from build123d import *

# Parameters (mm, degrees)
F0_R     = 20
F1_DEPTH = 17
F2_R     = 5
F3_DEPTH = 30.001
F4_DEPTH = 12.5
F0_R_2   = 5
F5_DEPTH = 14.5


# Not quite as in the source:
# - a feature names something its author has since deleted; it is built from what else it names


with BuildPart() as f1:
    # F0 (on Front) → F1 (new body, symmetric)
    with BuildSketch(Plane.XZ):
        with BuildLine():
            ThreePointArc((-22.5, 19.843134833), (-10.6066017178, -28.0624304008), (30, 0))
            ThreePointArc((30, 0), (28.0624304008, 10.6066017178), (22.5, 19.843134833))
            ThreePointArc((22.5, 19.843134833), (0, 30), (-22.5, 19.843134833))
        make_face()
        Circle(F0_R, mode=Mode.SUBTRACT)
    extrude(amount=F1_DEPTH, both=True)

    # F2 (on Right) → F3 (cut, through all)
    with BuildSketch(Plane.YZ):
        Circle(F2_R)
    extrude(amount=F3_DEPTH, mode=Mode.SUBTRACT)

    # F0 (on Front) → F4 (cut, symmetric)
    with BuildSketch(Plane.XZ):
        with BuildLine():
            ThreePointArc((6, 79.5607177772), (0, 78.5), (-6, 79.5607177772))
            Line((-6, 79.5607177772), (-6, 73.6))
            Line((-6, 73.6), (6, 73.6))
            Line((6, 73.6), (6, 79.5607177772))
        make_face()
    extrude(amount=F4_DEPTH, both=True, mode=Mode.SUBTRACT)

    # F0 (on Front) → F5 (join, symmetric)
    with BuildSketch(Plane.XZ):
        with BuildLine():
            ThreePointArc((-22.5, 19.843134833), (0, 30), (22.5, 19.843134833))
            Line((22.5, 19.843134833), (22.5, 166))
            Line((22.5, 166), (-22.5, 166))
            Line((-22.5, 166), (-22.5, 19.843134833))
        make_face()
        with BuildLine():
            ThreePointArc((-6, 79.5607177772), (-10.0312013239, 110.3396303997), (17.5, 96))
            ThreePointArc((17.5, 96), (14.3396303997, 85.9687986761), (6, 79.5607177772))
            Line((6, 79.5607177772), (6, 73.6))
            Line((6, 73.6), (-6, 73.6))
            Line((-6, 73.6), (-6, 79.5607177772))
        make_face(mode=Mode.SUBTRACT)
        with Locations((0, 140)):
            Circle(F0_R_2, mode=Mode.SUBTRACT)
    extrude(amount=F5_DEPTH, both=True)


solid = f1.part
Work out the finished part from the listing and answer in its coordinate system (mm). A direction names the side the tool comes from. Give positions to 0.01 mm unless a question says otherwise; leave off trailing zeros. Write each loop counter-clockwise with the first axis right and the second up, starting at its lowest first coordinate (ties: lowest second). Pieces come first, ordered by that corner, then holes. Notation, with made-up numbers: (85.5, 43.5) - (114.5, 43.5) arc R8 ccw to (114.5, 58.5) - close; hole circle Ø2 at (-35.75, 10.25). An arc over 180 degrees is marked (long way). One line per item, written item: value. Start each with the question number.
1. Consider probe 1 along Z at (x, y) = (0, 1); probe 2 along Y at (x, z) = (27, 0); probe 3 along Z at (x, y) = (5.5, 2). Determine where each line is inside the solid, lowest interval first.
2. For faces 4 (the flat face through (20, -17, -6)), 5 (the cylindrical face through (25, -5, 0)), 6 (the flat face through (-6, 0, 77)), 7 (the flat face through (22.5, 0, 92)), determine the directions among +Z, -Z, +X, -X, +Y, -Y from which every point of the face is accessible in a straight line to the end or side of a thin tool.
3. Find section D-D (z = 96). Write down the section's boundary in (x, y).
4. For a pull along X with two mould halves and no side action, classify faces 1 (the flat face through (20, 17, -6)), 2 (the flat face through (6, 0, 77)), 3 (the flat face through (-22.5, 0, 94)) as +X half, -X half, draft (parallel to the pull), parting line (faces both ways), or undercut.
5. Find section A-A (z = 0). Write down the section's boundary in (x, y).
6. Given pin 1 (4 mm diameter, centred on x = 5.5, z = 59.5, fed in from +Y); pin 2 (5 mm diameter, centred on y = -5.5, z = 28, fed in from -X); pin 3 (11.5 mm diameter, centred on x = 0, z = 140, fed in from -Y), each flat-ended and moving along its own axis, determine where each tip first touches the part or whether it passes through.
7. Find section B-B (x = 0). Write down the section's boundary in (y, z), then the cut area to 3 significant figures.
8. Find section C-C (y = 7). Write down the section's boundary in (x, z), then the cut area to 3 significant figures.
Geometry results:
1. probe 1: -30 to -20, 20 to 73.6, 113.5 to 135, 145 to 166
1. probe 2: -17 to -5, 5 to 17
1. probe 3: -29.49 to -19.23, 19.23 to 73.6, 112.61 to 166
2. face 4: +Z, -Z, +X, -X, -Y
2. face 5: +X
2. face 6: +Y, -Y
2. face 7: +Z, +X, +Y, -Y
3. outline: (-22.5, -14.5) - (-17.5, -14.5) - (-17.5, 14.5) - (-22.5, 14.5) - close; (17.5, -14.5) - (22.5, -14.5) - (22.5, 14.5) - (17.5, 14.5) - close
4. face 1: draft
4. face 2: undercut
4. face 3: -X half
5. outline: (-30, -17) - (-20, -17) - (-20, 17) - (-30, 17) - close; (20, -17) - (30, -17) - (30, -5) - (20, -5) - close; (20, 5) - (30, 5) - (30, 17) - (20, 17) - close
6. pin 1: y = 14.5
6. pin 2: x = -22.5
6. pin 3: y = -14.5
7. outline: (-17, -30) - (17, -30) - (17, -20) - (-17, -20) - close; (-17, 20) - (17, 20) - (17, 30) - (14.5, 30) - (14.5, 73.6) - (-14.5, 73.6) - (-14.5, 30) - (-17, 30) - close; (-14.5, 113.5) - (14.5, 113.5) - (14.5, 135) - (-14.5, 135) - close; (-14.5, 145) - (14.5, 145) - (14.5, 166) - (-14.5, 166) - close
7. area: 3,180 mm2
8. outline: (-22.5, 19.84) arc R30 ccw (long way) to (22.5, 19.84) - (22.5, 166) - (-22.5, 166) - close; hole circle Ø40 at (0, 0); hole (-6, 73.6) - (6, 73.6) - (6, 79.56) arc R17.5 ccw (long way) to (-6, 79.56) - close; hole circle Ø10 at (0, 140)
8. area: 6,730 mm2
